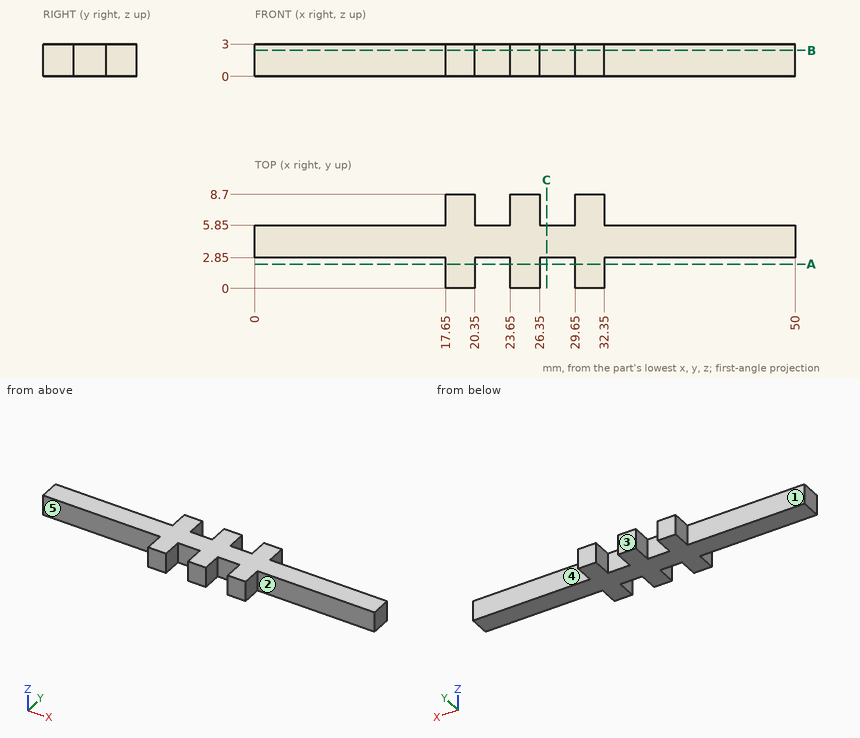
Design review of the part shown in the three views and the two pictorial views. Dimensions are in mm from the part's minimum x, y and z. A direction names the side the tool comes from. Give positions to 0.01 mm unless a question says otherwise; leave off trailing zeros. Write each loop counter-clockwise with the first axis right and the second up, starting at its lowest first coordinate (ties: lowest second). Pieces come first, ordered by that corner, then holes. Notation, with made-up numbers: (88, 0.25) -> (119, 0.25) arc R19 cw to (119, 22.25) -> close; hole circle Ø2 at (77.5, -14.75). An arc over 180 degrees is marked (long way). Answer in a Markdown table with one row per item.
1) Add section B-B on z = 2.4. State the section outline as (x, y) points, plus the area to 3 significant figures.
Worked answers:
| item | result |
|---|---|
| outline | (0, 2.85) -> (17.65, 2.85) -> (17.65, 0) -> (20.35, 0) -> (20.35, 2.85) -> (23.65, 2.85) -> (23.65, 0) -> (26.35, 0) -> (26.35, 2.85) -> (29.65, 2.85) -> (29.65, 0) -> (32.35, 0) -> (32.35, 2.85) -> (50, 2.85) -> (50, 5.85) -> (32.35, 5.85) -> (32.35, 8.7) -> (29.65, 8.7) -> (29.65, 5.85) -> (26.35, 5.85) -> (26.35, 8.7) -> (23.65, 8.7) -> (23.65, 5.85) -> (20.35, 5.85) -> (20.35, 8.7) -> (17.65, 8.7) -> (17.65, 5.85) -> (0, 5.85) -> close |
| area | 196 mm² |
2) Add section A-A on y = 2.25. State the section outline as (x, z) points.
Worked answers:
| item | result |
|---|---|
| outline | (17.65, 0) -> (20.35, 0) -> (20.35, 3) -> (17.65, 3) -> close; (23.65, 0) -> (26.35, 0) -> (26.35, 3) -> (23.65, 3) -> close; (29.65, 0) -> (32.35, 0) -> (32.35, 3) -> (29.65, 3) -> close |
3) Clearance check with flat-ended pins moving along their axes: P1, Ø1.5, axis at x = 37, z = 1, coming from the +Y side; P2, Ø1.4, axis at y = 7.5, z = 2, coming from the -X side; P3, Ø1.4, axis at y = 7.5, z = 2, coming from the +X side. State where each tip first meets the part, or that it passes through.
Worked answers:
| item | result |
|---|---|
| P1 | y = 5.85 |
| P2 | x = 17.65 |
| P3 | x = 32.35 |
4) Tool access review of the marked faces 1, 2, 3, 4 and 5: name each direction out of +Z, -Z, +X, -X, +Y, -Y from which nothing blocks a thin tool from reaching the whole face with its end or side.
Worked answers:
| item | result |
|---|---|
| face 1 | +Z, -Z, -X, +Y |
| face 2 | +Z, -Z, +X, -Y |
| face 3 | +Z, -Z, +X, -X, +Y |
| face 4 | +Z, -Z, +X, +Y |
| face 5 | +Z, -Z, -X, -Y |
5) For L1, parallel to X at y = 0.75, z = 1.8; L2, parallel to Y at x = 3, z = 1.35, list the stretches that pass through material, from the lowest coordinate up. Write a range as [from, to].
Worked answers:
| item | result |
|---|---|
| L1 | [17.65, 20.35], [23.65, 26.35], [29.65, 32.35] |
| L2 | [2.85, 5.85] |
6) Add section C-C on x = 27. State the section outline as (y, z) points.
Worked answers:
| item | result |
|---|---|
| outline | (2.85, 0) -> (5.85, 0) -> (5.85, 3) -> (2.85, 3) -> close |
